The drawing under review shows one solid part. Ordinate dimensions are in mm from its lowest x, y, z. Coordinates: 2 decimals unless noted, no trailing zeros. Loops run counter-clockwise (first coordinate to the right, second up) from the corner with the lowest first, then second, coordinate; pieces in that order, holes last. Notation, with made-up numbers: M 20.5,76.5 L 58.5,76.5 A6 cw 58.5,86.5 Z; hole C 1,51 d2. An arc over 180 degrees is marked long. Return JSON: item names as keys, results as strings.
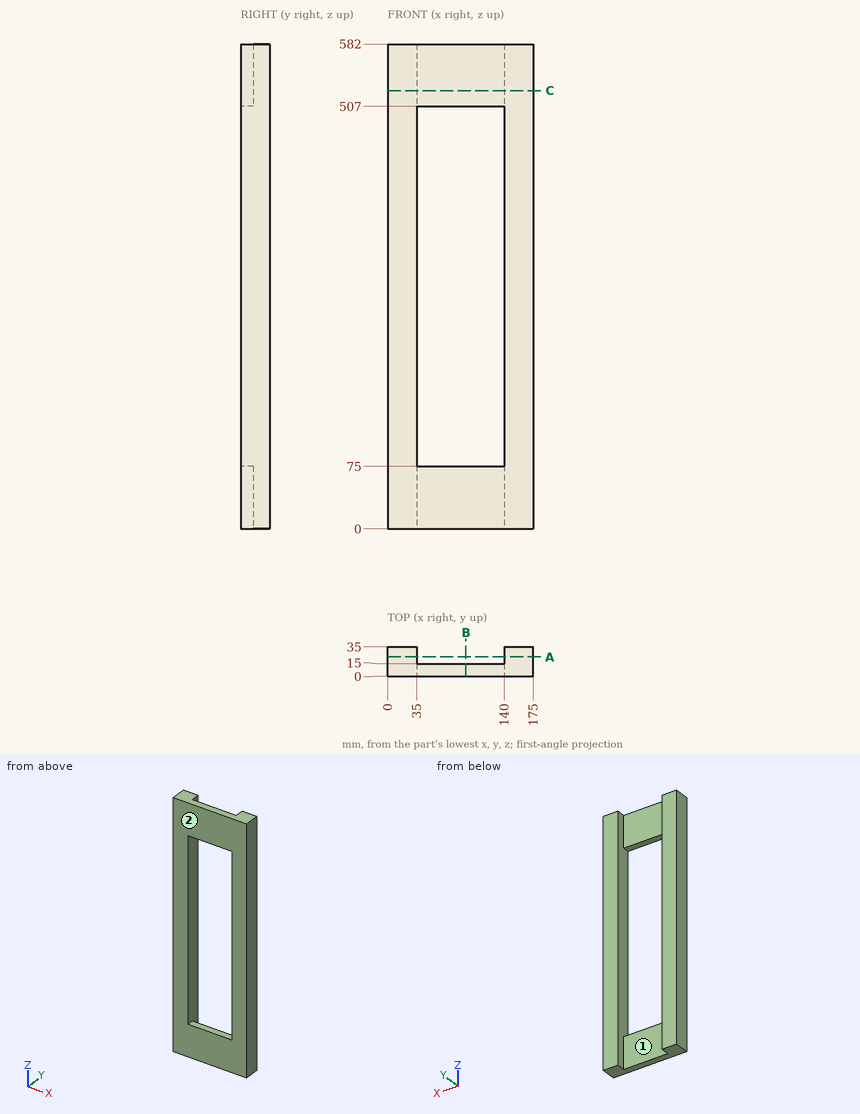
1. Add section A-A on y = 23. Give the boundary of the cut face in (x, z).
Check values:
{"outline": "M 0,0 L 35,0 L 35,582 L 0,582 Z; M 140,0 L 175,0 L 175,582 L 140,582 Z"}
2. Insertion check: pin 1 Ø22.5 at (x, z) = (84.5, 20.5) entering from +Y. The pin has a flat end and moves straight along its axis. Give the tip position at first contact, or say it passes through.
Check values:
{"pin 1": "y = 15"}
3. Add section C-C on z = 526. Give the boundary of the cut face in (x, y), plus the area to 4 significant figures.
Check values:
{"outline": "M 0,0 L 175,0 L 175,35 L 140,35 L 140,15 L 35,15 L 35,35 L 0,35 Z", "area": "4,025 mm²"}
4. The part is to be moulded in two halves that separate along X. For the marked faces 1 and 2, say which applies: released by +X, released by -X, zero draft, split by the parting line, or undercut.
Check values:
{"face 1": "undercut", "face 2": "zero draft"}
5. Add section B-B on x = 94. Give the boundary of the cut face in (y, z).
Check values:
{"outline": "M 0,0 L 15,0 L 15,75 L 0,75 Z; M 0,507 L 15,507 L 15,582 L 0,582 Z"}
6. To check wall thickness, follow line 1 (X direction, y = 33.5, z = 83); line 2 (Z direction, x = 42, y = 7); line 3 (Y direction, x = 114, z = 543.5). State the ranges of each line that lie inside material, in increasing order.
Check values:
{"line 1": "0 to 35, 140 to 175", "line 2": "0 to 75, 507 to 582", "line 3": "0 to 15"}
